Geometry check sheet. Reference: drawing and pictorial views, mm from the part's lowest x, y, z. Give positions to 0.01 mm unless a question says otherwise; leave off trailing zeros. Write each loop counter-clockwise with the first axis right and the second up, starting at its lowest first coordinate (ties: lowest second). Pieces come first, ordered by that corner, then holes. Notation, with made-up numbers: (-0.75, 40.25) - (6.25, 40.25) arc R34 ccw to (6.25, 76.25) - close; hole circle Ø3 at (-23.5, -2). An arc over 180 degrees is marked (long way). Put each result on its own line as item: value.
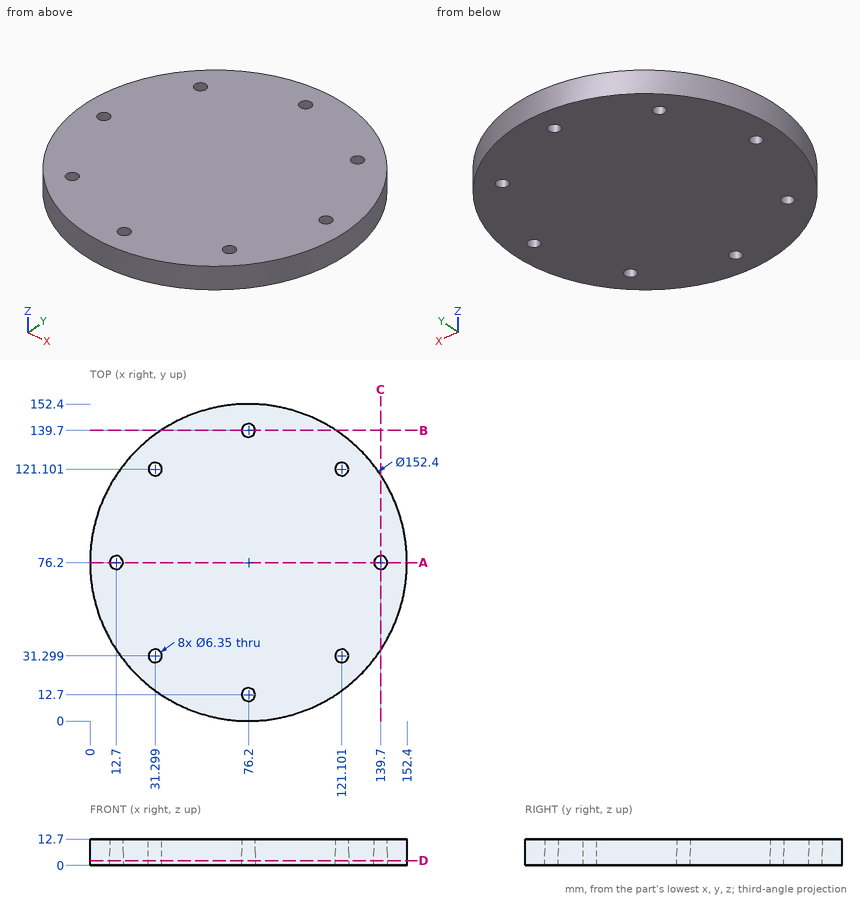
Q1. Section check B-B, the plane y = 139.7. Record the cut outline in (x, z) (1 decimal), plus the area to 3 significant figures.
Answers follow:
outline: (34.1, 0) - (73, 0) - (73, 12.7) - (34.1, 12.7) - close; (79.4, 0) - (118.3, 0) - (118.3, 12.7) - (79.4, 12.7) - close
area: 989 mm2
Q2. Go/stop test with flat-tipped pins: pin 1 Ø4 at (y, z) = (82.5, 7) entering from +X; pin 2 Ø4 at (x, y) = (139.7, 76.2) entering from +Z; pin 3 Ø10 at (x, y) = (31.3, 121.1) entering from +Z; pin 4 Ø6 at (x, z) = (72.5, 10.5) entering from -Y. Record where each tip stops, or that it passes through.
Answers follow:
pin 1: stops at x = 152.28
pin 2: passes through
pin 3: stops at z = 12.7
pin 4: stops at y = 0
Q3. Section check D-D, the plane z = 2.25. Give the number of separate pieces and of enclosed holes in the cut face, plus the area to 3 significant figures.
Answers follow:
separate pieces: 1
enclosed holes: 8
area: 18,000 mm2
Q4. Scan lines: line 1 along X through (y, z) = (76, 4); line 2 along Y through (x, z) = (32.5, 6) (1 decimal); line 3 along Y through (x, z) = (12, 7.5) (1 decimal). Record each from-to range of solid material in increasing order.
Answers follow:
line 1: x = 0 to 9.53, 15.87 to 136.53, 142.87 to 152.4
line 2: y = 13.8 to 28.4, 34.2 to 118.2, 124 to 138.6
line 3: y = 35.2 to 73.1, 79.3 to 117.2
Q5. Section check A-A, the plane y = 76.2. Record the cut outline in (x, z) (1 decimal).
Answers follow:
outline: (0, 0) - (9.5, 0) - (9.5, 12.7) - (0, 12.7) - close; (15.9, 0) - (136.5, 0) - (136.5, 12.7) - (15.9, 12.7) - close; (142.9, 0) - (152.4, 0) - (152.4, 12.7) - (142.9, 12.7) - close
